```python
from build123d import *

# Parameters (mm, degrees)
BOSS_EXTRUDE1_DEPTH      = 22.225
M6_CLEARANCE_HOLE1_D     = 6.5278
M6_CLEARANCE_HOLE1_DEPTH = 63.5
M6_CLEARANCE_HOLE2_D     = 6.5278
M6_CLEARANCE_HOLE2_DEPTH = 63.5
FILLET1_R                = 4.7625


with BuildPart() as part:
    # Sketch1 → Boss-Extrude1 (new body)
    with BuildSketch(Plane(origin=(11.1125, 0, 0), x_dir=(0, 0, -1), z_dir=(1, 0, 0))):
        with BuildLine():
            Line((-4.767789963, 58.742792373), (-4.767789963, 4.767792373))
            Line((-4.767789963, 4.767792373), (-58.742789963, 4.767792373))
            ThreePointArc((-58.742789963, 4.767792373), (-62.110386009, 3.372888418), (-63.505289963, 0.005292373))
            Line((-63.505289963, 0.005292373), (-0.005289963, 0.005292373))
            Line((-0.005289963, 0.005292373), (-0.005289963, 63.505292373))
            ThreePointArc((-0.005289963, 63.505292373), (-3.372886009, 62.110388418), (-4.767789963, 58.742792373))
        make_face()
    extrude(amount=-BOSS_EXTRUDE1_DEPTH)

    # M6 Clearance Hole1
    with Locations(Plane.XZ.offset(-0.005292373)):
        with Locations((0, 19.055289963), (0, 44.455289963)):
            Hole(M6_CLEARANCE_HOLE1_D / 2, depth=M6_CLEARANCE_HOLE1_DEPTH)

    # M6 Clearance Hole2
    with Locations(Plane(origin=(0, 0, 0.005289963), x_dir=(-1, 0, 0), z_dir=(0, 0, -1))):
        with Locations((0, 19.055292373), (0, 44.455292373)):
            Hole(M6_CLEARANCE_HOLE2_D / 2, depth=M6_CLEARANCE_HOLE2_DEPTH)

    # Fillet1
    fillet1_edges = [part.edges().sort_by_distance(p)[0] for p in [
        (0, 4.767792373, 4.767789963),
    ]]
    fillet(fillet1_edges, radius=FILLET1_R)


solid = part.part
```
Part model, mm, in its own coordinate system. A direction names the side the tool comes from. Round coordinates to 2 decimals unless told otherwise and drop trailing zeros. Order: outer loops, then holes, each group sorted by start corner. A loop starts at its lowest first (then second) coordinate and runs counter-clockwise, first axis right, second up. Notation, with made-up numbers: M -25.75,29.25 L -5.75,29.25 A22 cw -5.75,59.25 Z; hole C 39,7.5 d8. An arc over 180 degrees is marked long. Answer in a Markdown table with one row per item. Add a question column.
Q1. Pin check, flat tips, straight feed: pin 1 (1.5 mm diameter, centred on x = -3, y = 55, fed in from +Z); pin 2 (2 mm diameter, centred on x = 2, y = 42.5, fed in from -Z); pin 3 (12 mm diameter, centred on x = 4.5, z = 17, fed in from +Y). Stop position of each tip, or through.
Q2. Wall check: L1, parallel to Z at x = 0, y = 3.4; L2, parallel to Y at x = 0, z = 1.85; L3, parallel to Z at x = 0, y = 3.8. Give the ranges that are in metal, low to high. Write a range as from..to.
Q3. Cut at C-C on x = -7. Give the cut face in (y, z) (1 decimal), and give its area (3 significant figures).
Q4. Cut at D-D on y = 25. Give the cut face in (x, z), and give its area (3 significant figures).
Q5. 3-axis set-ups, long thin cutter, end or side, ignore diameter. For faces 1 (the face through (0, 4.768, 34)), 2 (the face through (0.425, 2.42, 47.691)): which of +Z, -Z, +X, -X, +Y, -Y reach the whole face in a straight line?
Q6. Cut at A-A on x = 0. Give the cut face in (y, z) (1 decimal), and give its area (3 significant figures).
Q7. Mould opens along X. For faces 3 (the face through (-2.59, 42.47, 2.42)), 4 (the face through (-11.112, 4, 18)), 5 (the face through (0, 0.005, 32)) say: +X half, -X half, draft (parallel to the pull), parting line (faces both ways), or undercut.
Q8. Cut at B-B on z = 46. Give the cut face in (x, y).
Established:
| question | item | result |
|---|---|---|
| 1 | pin 1 | stops at z = 4.77 |
| 1 | pin 2 | stops at z = 0.01 |
| 1 | pin 3 | stops at y = 4.77 |
| 2 | L1 | z = 0.01..15.79, 22.32..41.19, 47.72..62.08 |
| 2 | L2 | y = 0.01..15.79, 22.32..41.19, 47.72..63.13 |
| 2 | L3 | z = 0.01..15.79, 22.32..41.19, 47.72..61.62 |
| 3 | outline | M 0,0 L 63.5,0 A4.8 ccw 58.7,4.8 L 9.5,4.8 A4.8 cw 4.8,9.5 L 4.8,58.7 A4.8 ccw 0,63.5 Z |
| 3 | area | 577 mm2 |
| 4 | outline | M -11.11,0.01 L 11.11,0.01 L 11.11,4.77 L -11.11,4.77 Z |
| 4 | area | 106 mm2 |
| 5 | face 1 | +Z, +X, -X, +Y |
| 5 | face 2 | +Y, -Y |
| 6 | outline | M 0,0 L 15.8,0 L 15.8,4.8 L 9.5,4.8 A4.8 cw 4.8,9.5 L 4.8,15.8 L 0,15.8 Z; M 0,22.3 L 4.8,22.3 L 4.8,41.2 L 0,41.2 Z; M 0,47.7 L 4.8,47.7 L 4.8,58.7 A4.8 ccw 0,63.5 Z; M 22.3,0 L 41.2,0 L 41.2,4.8 L 22.3,4.8 Z; M 47.7,0 L 63.5,0 A4.8 ccw 58.7,4.8 L 47.7,4.8 Z |
| 6 | area | 453 mm2 |
| 7 | face 3 | undercut |
| 7 | face 4 | -X half |
| 7 | face 5 | draft |
| 8 | outline | M -11.11,0.01 L -2.88,0.01 L -2.88,4.77 L -11.11,4.77 Z; M 2.88,0.01 L 11.11,0.01 L 11.11,4.77 L 2.88,4.77 Z |
